from build123d import *

# Parameters (mm, degrees)
SKETCH1_R           = 4.699
BOSS_EXTRUDE1_DEPTH = 6.223
SKETCH2_R           = 5.2324
BOSS_EXTRUDE2_DEPTH = 21.2852
SKETCH3_R           = 3.937
BOSS_EXTRUDE3_DEPTH = 31.9024


with BuildPart() as part:
    # Sketch1 → Boss-Extrude1 (new body)
    with BuildSketch(Plane.XY):
        with BuildLine():
            Line((27.839647422, -1.363090318), (24.347147422, 24.925909682))
            ThreePointArc((24.347147422, 24.925909682), (16.183361565, 40.166897281), (0, 46.252446639))
            ThreePointArc((0, 46.252446639), (-16.183361565, 40.166897281), (-24.347147422, 24.925909682))
            Line((-24.347147422, 24.925909682), (-27.839647422, -1.363090318))
            ThreePointArc((-27.839647422, -1.363090318), (-39.463090318, -10.260352578), (-48.360352578, 1.363090318))
            Line((-48.360352578, 1.363090318), (-44.867852578, 27.652090318))
            ThreePointArc((-44.867852578, 27.652090318), (-43.214104666, 32.038713591), (-39.794788795, 35.245834553))
            Line((-39.794788795, 35.245834553), (-15.873370018, 49.099758822))
            ThreePointArc((-15.873370018, 49.099758822), (0, 53.364446639), (15.873370018, 49.099758822))
            Line((15.873370018, 49.099758822), (39.794788795, 35.245834553))
            ThreePointArc((39.794788795, 35.245834553), (43.214104666, 32.038713591), (44.867852578, 27.652090318))
            Line((44.867852578, 27.652090318), (48.360352578, 1.363090318))
            ThreePointArc((48.360352578, 1.363090318), (39.463090318, -10.260352578), (27.839647422, -1.363090318))
        make_face()
        with Locations((34.6075, 26.289)):
            Circle(SKETCH1_R, mode=Mode.SUBTRACT)
        with Locations(Location((-34.6075, 26.289, 0), (0, 0, 180))):
            Circle(SKETCH1_R, mode=Mode.SUBTRACT)
    extrude(amount=BOSS_EXTRUDE1_DEPTH)

    # Sketch2 → Boss-Extrude2 (add)
    with BuildSketch(Plane.XY.offset(6.223)):
        with Locations((38.1, 0)):
            Circle(SKETCH2_R)
    boss_extrude2 = extrude(amount=BOSS_EXTRUDE2_DEPTH)

    # Mirror1: Boss-Extrude2 across plane
    add(boss_extrude2.mirror(Plane(origin=(0, 0, 0), x_dir=(0, 0, 1), z_dir=(1, 0, 0))))

    # Sketch3 → Boss-Extrude3 (add)
    with BuildSketch(Plane(origin=(0, 0, 0), x_dir=(-1, 0, 0), z_dir=(0, 0, -1))):
        with Locations(Location((38.1, 0, 0), (0, 0, 180))):
            Circle(SKETCH3_R)
    boss_extrude3 = extrude(amount=BOSS_EXTRUDE3_DEPTH)

    # Mirror2: Boss-Extrude3 across plane
    add(boss_extrude3.mirror(Plane(origin=(0, 0, 0), x_dir=(0, 0, 1), z_dir=(1, 0, 0))))


solid = part.part
For this review, take the finished solid that the model builds, in its own axes (mm). A direction names the side the tool comes from. Coordinates: 2 decimals unless noted, no trailing zeros. Loops run counter-clockwise (first coordinate to the right, second up) from the corner with the lowest first, then second, coordinate; pieces in that order, holes last. Notation, with made-up numbers: (5.5, 43.5) - (24.5, 43.5) arc R20 cw to (24.5, 66.5) - close; hole circle Ø7 at (39, 31.25). An arc over 180 degrees is marked (long way). Use a Markdown table: item, result. Add a question column.
Item 1: For line 1 (Z direction, x = -29, y = 25); line 2 (X direction, y = -4, z = 23.5); line 3 (X direction, y = 7.5, z = 1), list the stretches that pass through material, from the lowest coordinate up.
Item 2: Tool access review of faces 4 (the face through (42.033, -0.173, -15.728)), 5 (the face through (-42.933, -2.004, 16.717)), 6 (the face through (-0.233, 53.364, 3.068)): name each direction out of +Z, -Z, +X, -X, +Y, -Y from which nothing blocks a thin tool from reaching the whole face with its end or side.
Item 3: Insertion check: pin 1 Ø10 at (x, y) = (13, 36.5) entering from +Z; pin 2 Ø10 at (x, y) = (32, 45.5) entering from -Z; pin 3 Ø8 at (y, z) = (36.5, 3.5) entering from +X. Each pin has a flat end and moves straight along its axis. Give the tip position at first contact, or say it passes through.
Item 4: We need section A-A (y = 20). Give the boundary of the cut face in (x, z), and give its area (3 significant figures).
Item 5: Mouldability with a two-part tool opening along X and no side actions: class faces 1 (the face through (43.18, 32.09, 3.07)), 2 (the face through (-46.64, 14.32, 3.07)), 3 (the face through (42.933, -2.004, 16.717)) as pulls with the +X half, pulls with the -X half, needs draft (parallel to the pull), parting line crosses it, or undercut.
Item 6: We need section C-C (z = 21.5). Give the boundary of the cut face in (x, y).
Item 7: We need section B-B (x = -37). Give the boundary of the cut face in (y, z), and give its area (3 significant figures).
Item 8: We need section D-D (y = 0). Give the boundary of the cut face in (x, z).
Results list:
| question | item | result |
|---|---|---|
| 1 | line 1 | z = 0 to 6.22 |
| 1 | line 2 | x = -41.47 to -34.73, 34.73 to 41.47 |
| 1 | line 3 | x = -47.55 to -26.66, 26.66 to 47.55 |
| 2 | face 4 | -Z |
| 2 | face 5 | +Z |
| 2 | face 6 | +Z, -Z, +Y |
| 3 | pin 1 | stops at z = 6.22 |
| 3 | pin 2 | stops at z = 0 |
| 3 | pin 3 | stops at x = 42.89 |
| 4 | outline | (-45.88, 0) - (-25, 0) - (-25, 6.22) - (-45.88, 6.22) - close; (25, 0) - (45.88, 0) - (45.88, 6.22) - (25, 6.22) - close |
| 4 | area | 260 mm^2 |
| 5 | face 1 | pulls with the +X half |
| 5 | face 2 | pulls with the -X half |
| 5 | face 3 | undercut |
| 6 | outline | circle Ø10.46 at (-38.1, 0); circle Ø10.46 at (38.1, 0) |
| 7 | outline | (-10.29, 0) - (-3.78, 0) - (-3.78, -31.9) - (3.78, -31.9) - (3.78, 0) - (22.24, 0) - (22.24, 6.22) - (5.12, 6.22) - (5.12, 27.51) - (-5.12, 27.51) - (-5.12, 6.22) - (-10.29, 6.22) - close; (30.33, 0) - (36.86, 0) - (36.86, 6.22) - (30.33, 6.22) - close |
| 7 | area | 702 mm^2 |
| 8 | outline | (-48.45, 0) - (-42.04, 0) - (-42.04, -31.9) - (-34.16, -31.9) - (-34.16, 0) - (-27.66, 0) - (-27.66, 6.22) - (-32.87, 6.22) - (-32.87, 27.51) - (-43.33, 27.51) - (-43.33, 6.22) - (-48.45, 6.22) - close; (27.66, 0) - (34.16, 0) - (34.16, -31.9) - (42.04, -31.9) - (42.04, 0) - (48.45, 0) - (48.45, 6.22) - (43.33, 6.22) - (43.33, 27.51) - (32.87, 27.51) - (32.87, 6.22) - (27.66, 6.22) - close |
